The listing builds one solid part. Answer for the finished solid, in the listing's coordinates (mm). Give positions to 0.01 mm unless a question says otherwise; leave off trailing zeros. Loops run counter-clockwise (first coordinate to the right, second up) from the corner with the lowest first, then second, coordinate; pieces in that order, holes last. Notation, with made-up numbers: M 18,57.5 L 54,57.5 A22 ccw 54,95.5 Z; hole C 58.5,12.5 d10. An arc over 180 degrees is marked long. One line per item, written item: value. Start each with the question number.
Q1. A cutting plane is placed at D-D, the plane x = 70.5. Determine the outline of the cut face in (y, z) (3 decimals).
Q2. A cutting plane is placed at A-A, the plane x = 266.7. Determine the outline of the cut face in (y, z) (1 decimal).
Q3. Flat-ended cylindrical pins translate along their axes: pin 1 (1.6 mm diameter, centred on y = 10.5, z = 2.5, fed in from +X); pin 2 (5.5 mm diameter, centred on x = -288.925, y = 0, fed in from +Z); pin 3 (1.6 mm diameter, centred on x = -247.5, z = 2.5, fed in from -Y) (3 decimals); pin 4 (1 mm diameter, centred on y = 10, z = 2, fed in from -X). Find the tip coordinate at first contact, or state that the pin passes through.
Q4. A cutting plane is placed at B-B, the plane y = 0. State how many separate pieces and enclosed holes the cut face has, and give its area (3 significant figures).
Q5. Consider L1, parallel to X at y = -9.25, z = 2.65; L2, parallel to Y at x = 164.5, z = 0.4 (3 decimals); L3, parallel to Y at x = -246, z = 0.85 (3 decimals). Determine where each line is inside the solid, lowest interval first.
Q6. The mould has two halves that part along X. Classify faces 1 (the flat face through (-4, 0, 3.175)), 2 (the cylindrical face through (271.585, 0.215, 1.565)): +X half, -X half, draft (parallel to the pull), parting line (faces both ways), or undercut.
from build123d import *

# Parameters (mm, degrees)
SKETCH1_W           = 596.9
SKETCH1_H           = 16.51
BOSS_EXTRUDE1_DEPTH = 3.175
SKETCH3_W           = 37.846
SKETCH3_H           = 3.175
BOSS_EXTRUDE2_DEPTH = 3.175
SKETCH4_R           = 3.556
SKETCH4_R_2         = 4.8895
CUT_EXTRUDE1_DEPTH  = 299.685667592


with BuildPart() as part:
    # Sketch1 → Boss-Extrude1 (new body)
    with BuildSketch(Plane.XY):
        Rectangle(SKETCH1_W, SKETCH1_H)
    extrude(amount=BOSS_EXTRUDE1_DEPTH)

    # Sketch3 → Boss-Extrude2 (add)
    with BuildSketch(Plane(origin=(0, 8.255, 0), x_dir=(1, 0, 0), z_dir=(0, 1, 0))):
        with Locations((-199.093666667, -1.5875)):
            Rectangle(SKETCH3_W, SKETCH3_H)
        with Locations((-99.610333333, -1.5875)):
            Rectangle(SKETCH3_W, SKETCH3_H)
        with Locations((-0.127, -1.5875)):
            Rectangle(SKETCH3_W, SKETCH3_H)
        with Locations((99.483333333, -1.5875)):
            Rectangle(SKETCH3_W, SKETCH3_H)
        with Locations((198.966666751, -1.5875)):
            Rectangle(SKETCH3_W, SKETCH3_H)
    boss_extrude2 = extrude(amount=BOSS_EXTRUDE2_DEPTH)

    # Mirror1: Boss-Extrude2 across plane
    add(boss_extrude2.mirror(Plane.ZX))

    # Sketch4 → Cut-Extrude1 (cut, through all)
    with BuildSketch(Plane(origin=(0, 0, 0), x_dir=(-1, 0, 0), z_dir=(0, 0, -1))):
        with Locations((-288.925, 0)):
            Circle(SKETCH4_R)
        with Locations((-244.475, 0)):
            Circle(SKETCH4_R)
        with Locations((-266.7, 0)):
            Circle(SKETCH4_R_2)
    cut_extrude1 = extrude(amount=-CUT_EXTRUDE1_DEPTH, mode=Mode.SUBTRACT)

    # Mirror2: Cut-Extrude1 across plane
    add(cut_extrude1.mirror(Plane(origin=(0, 0, 0), x_dir=(0, 0, 1), z_dir=(1, 0, 0))), mode=Mode.SUBTRACT)


solid = part.part
Answer block:
1. outline: M -8.255,0 L 8.255,0 L 8.255,3.175 L -8.255,3.175 Z
2. outline: M -8.3,0 L -4.9,0 L -4.9,3.2 L -8.3,3.2 Z; M 4.9,0 L 8.3,0 L 8.3,3.2 L 4.9,3.2 Z
3. pin 1: x = 217.89
3. pin 2: through
3. pin 3: y = -8.255
3. pin 4: x = -218.02
4. separate pieces: 7
4. enclosed holes: 0
4. area: 1,740 mm^2
5. L1: -218.02 to -180.17, -118.53 to -80.69, -19.05 to 18.8, 80.56 to 118.41, 180.04 to 217.89
5. L2: -8.255 to 8.255
5. L3: -8.255 to -3.212, 3.212 to 8.255
6. face 1: draft
6. face 2: undercut
